Autodesk Inventor part; units mm, degrees
ref_plane "YZ Plane" through (0, 0, 0) normal (1, 0, 0) x (0, 1, 0)
ref_plane "XZ Plane" through (0, 0, 0) normal (0, 1, 0) x (-1, 0, 0)
ref_plane "XY Plane" through (0, 0, 0) normal (0, 0, 1) x (1, 0, 0)
sketch "Sketch1" plane through (0, 0, 0) normal (1, 0, 0) x (0, 1, 0)
  circle A0 centre (0, 0) radius 4
  circle A1 centre (0, 0) radius 5
  dimension "d0" = 8
  dimension "d1" = 10
extrude "Extrusion1" add sketch "Sketch1" along normal blind 10
sketch "Sketch2" plane through (10, 0, 0) normal (1, 0, 0) x (0, 0, -1)
  circle A0 centre (0, 0) radius 4
  circle A1 centre (0, 0) radius 5
extrude "Extrusion2" add sketch "Sketch2" along normal blind 10 contours A0 | A1
sketch "Sketch3" plane through (20, 0, 0) normal (1, 0, 0) x (0, 0, -1)
  circle A0 centre (0, 0) radius 10
  dimension "d6" = 20
loft "Loft1" add profiles "Sketch2", "Sketch3" contours A0 | A1 / all
sketch "Sketch4" plane through (0, 0, 0) normal (0, 0, 1) x (1, 0, 0)
  line L0 (10, 5) -> (10, -5)
  line L1 (20, 10) -> (20, -10)
  line L2 (-4, 0) -> (24, 0)
  line L3 (20, 2.5) -> (17, 0)
  line L4 (20, 10) -> (20, -10)
  line L5 (20, -2.5) -> (17, 0)
  line L6 (20, 2.5) -> (20, -2.5)
  point P0 (0, 0)
  dimension "d11" = 5
  dimension "d12" = 3
extrude "Extrusion3" cut sketch "Sketch4" along normal mid plane 20
sketch "Sketch5" plane through (0, 0, 0) normal (0, 1, 0) x (-1, 0, 0)
  line L0 (-10, -5) -> (-10, 5)
  line L1 (0, -5) -> (0, 5)
  circle A0 centre (-5, 0) radius 2
  line L2 (0, 0) -> (-10, 0)
  dimension "d15" = 4
  dimension "d16" = 5
extrude "Extrusion4" cut sketch "Sketch5" against normal up to next
thread "Thread1"
properties part number "Hand" material "PC/ABS Plastic"
Here's how the part is built. I have some questions about the finished solid (model axes, mm). A direction names the side the tool comes from. Coordinates: 2 decimals unless noted, no trailing zeros. Loops run counter-clockwise (first coordinate to the right, second up) from the corner with the lowest first, then second, coordinate; pieces in that order, holes last. Notation, with made-up numbers: (80.25, 58.5) -> (86.25, 58.5) arc R21 ccw to (86.25, 93.5) -> close; hole circle Ø9 at (-1, -35.5). An arc over 180 degrees is marked (long way). Use one line per item in the form item = value. Start each with the question number.
(1) Please list where these lines run through material, in increasing order: line 1 along Y through (x, z) = (7.75, 0); line 2 along Z through (x, y) = (2, 2.5).
(2) If we section it at A-A (z = 0): Please give me the cut outline in (x, y).
(3) We'd pull the mould along Y, two halves only. Please class faces 4 (the face through (11.74, 1.76, -5.6)), 5 (the face through (20, 5, 0)), 6 (the face through (18.521, 1.267, -0.136)): pulls with the +Y half, pulls with the -Y half, needs draft (parallel to the pull), parting line crosses it, or undercut.
(4) Will these pins go through, and if not, where does the flat tip stop? pin 1 (10 mm diameter, centred on x = 10, y = 7, fed in from -Z); pin 2 (5 mm diameter, centred on y = -6.5, z = 7.5, fed in from -X); pin 3 (5 mm diameter, centred on x = 7, z = -6.5, fed in from -Y).
(5) On a 3-axis mill with a long thin cutter (end or side, diameter ignored), from which of +Z, -Z, +X, -X, +Y, -Y can I reach the whole of each face in a straight line? I mean faces 1 (the face through (10, 0, 0)), 2 (the face through (20, -5, 0)), 3 (the face through (6.998, -4.221, 0.088)). Say none if no direction works.
(6) If we section it at D-D (x = 14.25): Please give me the cut outline in (y, z) (3 decimals), then the cut area to 3 significant figures.
(7) If we section it at C-C (x = 5): Please give me the cut outline in (y, z), then the cut area to 3 significant figures.
(8) If we section it at B-B (x = 2): Please give me the cut outline in (y, z).
Verdict:
q1.line_1 = -5 to -4, 4 to 5
q1.line_2 = -4.33 to -3.12, 3.12 to 4.33
q2.outline = (0, -5) -> (3, -5) -> (3, -4) -> (0, -4) -> close; (0, 4) -> (10, 4) -> (10, -4) -> (7, -4) -> (7, -5) -> (10, -5) -> (20, -10) -> (20, -2.5) -> (17, 0) -> (20, 2.5) -> (20, 10) -> (10, 5) -> (0, 5) -> close
q3.face_4 = parting line crosses it
q3.face_5 = needs draft
q3.face_6 = undercut
q4.pin_1 = -5.81
q4.pin_2 = 14.85
q4.pin_3 = -3
q5.face_1 = -X
q5.face_2 = +Z, -Z, +X, +Y, -Y
q5.face_3 = -Y
q6.outline = circle Ø14.25 at (0, 0)
q6.area = 159 mm²
q7.outline = (-4.58, -2) arc R5 ccw (long way) to (-4.58, 2) -> (-3.46, 2) arc R4 cw (long way) to (-3.46, -2) -> close
q7.area = 24.1 mm²
q8.outline = circle Ø10 at (0, 0); hole circle Ø8 at (0, 0)
